For this review, use the dimensioned drawing (mm, ordinates from the lowest corner) and the shaded views. A direction names the side the tool comes from. Give positions to 0.01 mm unless a question says otherwise; leave off trailing zeros. Order: outer loops, then holes, each group sorted by start corner. A loop starts at its lowest first (then second) coordinate and runs counter-clockwise, first axis right, second up. Notation, with made-up numbers: (35.25, 29.5) - (69.25, 29.5) arc R32 ccw to (69.25, 64.5) - close; hole circle Ø6 at (-37.75, 21). An arc over 180 degrees is marked (long way). Use a Markdown table: item, result. Add a question column.
1) Clearance check with flat-ended pins moving along their axes: P1, Ø5, axis at x = 16, y = 50.5, coming from the +Z side; P2, Ø2, axis at y = 29, z = 12.5, coming from the -X side; P3, Ø1, axis at x = 45.5, z = 9, coming from the -Y side. State where each tip first meets the part, or that it passes through.
2) We need section C-C on x = 31.5. Write out the cut boundary in (y, z), then the cut area to 3 significant figures.
3) We need section A-A on x = 16.5. Write out the cut boundary in (y, z).
4) We need section D-D on y = 31.5. Write out the cut boundary in (x, z), then the cut area to 3 significant figures.
5) Machinability: for the marked faces 1, 2 and 3, which of the approach directions +Z, -Z, +X, -X, +Y, -Y give a long, thin tool a straight path to every point of the face, cutting with its end or side? Answer none if there is none.
6) We need section B-B on z = 13. Write out the cut boundary in (x, y).
7) Mouldability with a two-part tool opening along Y and no side actions: class the marked faces 4, 5, 6 and 7 as released by +Y, released by -Y, zero draft, split by the parting line, or undercut.
8) Wall thickness on L1, parallel to X at y = 53.5, z = 11.25 (1 decimal); L2, parallel to X at y = 48, z = 10.5; L3, parallel to Y at x = 16.5, z = 7.5: over which ranges is each line inside the solid? List them lowest first.
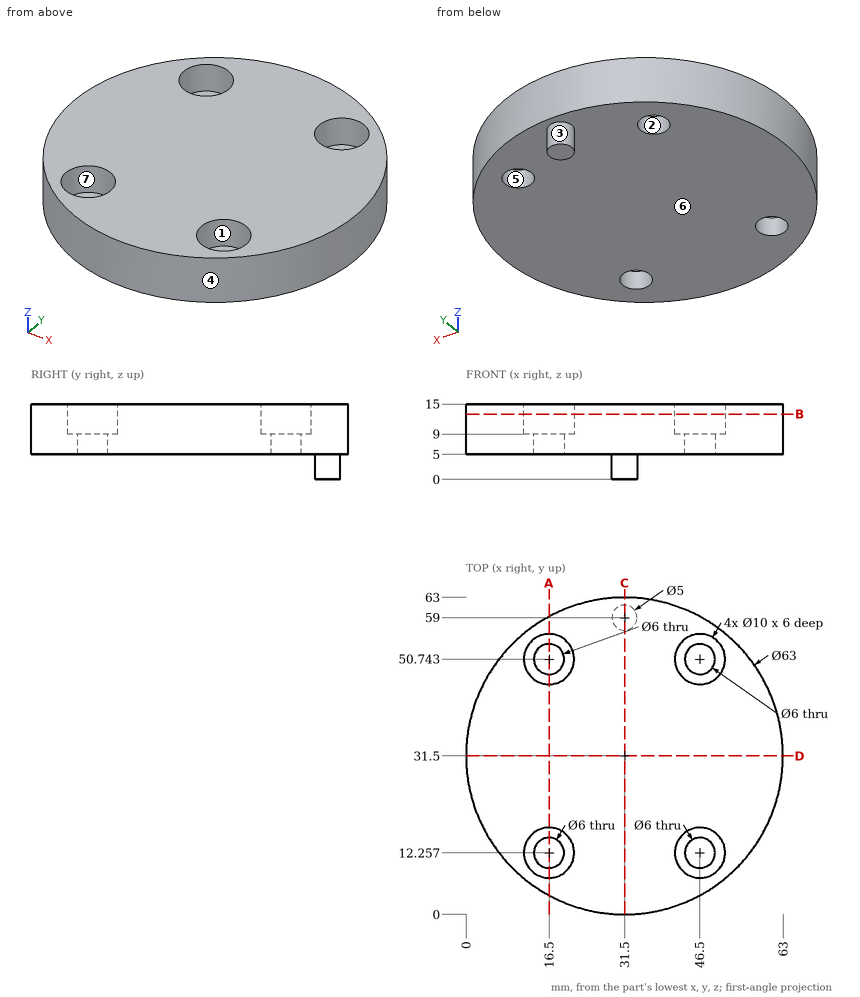
Checked values:
| question | item | result |
|---|---|---|
| 1 | P1 | z = 9 |
| 1 | P2 | x = 0.04 |
| 1 | P3 | y = 3.04 |
| 2 | outline | (0, 5) - (56.5, 5) - (56.5, 0) - (61.5, 0) - (61.5, 5) - (63, 5) - (63, 15) - (0, 15) - close |
| 2 | area | 655 mm² |
| 3 | outline | (3.8, 5) - (9.26, 5) - (9.26, 9) - (7.26, 9) - (7.26, 15) - (3.8, 15) - close; (15.26, 5) - (47.74, 5) - (47.74, 9) - (45.74, 9) - (45.74, 15) - (17.26, 15) - (17.26, 9) - (15.26, 9) - close; (53.74, 5) - (59.2, 5) - (59.2, 15) - (55.74, 15) - (55.74, 9) - (53.74, 9) - close |
| 4 | outline | (0, 5) - (63, 5) - (63, 15) - (0, 15) - close |
| 4 | area | 630 mm² |
| 5 | face 1 | +Z |
| 5 | face 2 | +Z, -Z |
| 5 | face 3 | -Z |
| 6 | outline | circle Ø63 at (31.5, 31.5); hole circle Ø10 at (16.5, 12.26); hole circle Ø10 at (16.5, 50.74); hole circle Ø10 at (46.5, 12.26); hole circle Ø10 at (46.5, 50.74) |
| 7 | face 4 | split by the parting line |
| 7 | face 5 | undercut |
| 7 | face 6 | zero draft |
| 7 | face 7 | undercut |
| 8 | L1 | 9 to 12.3, 20.7 to 42.3, 50.7 to 54 |
| 8 | L2 | 4.67 to 12.32, 20.68 to 42.32, 50.68 to 58.33 |
| 8 | L3 | 3.8 to 9.26, 15.26 to 47.74, 53.74 to 59.2 |
